from build123d import *

# Parameters (mm, degrees)
F1_DEPTH = 25.4
F2_W     = 19.05
F2_H     = 4.923508
F3_DEPTH = 25.4
F4_R     = 3.175
F5_DEPTH = 12.701
F6_R     = 3.175
F7_DEPTH = 25.4
F8_W     = 19.05
F8_H     = 19.05
F9_DEPTH = 6.35


with BuildPart() as f1:
    # F0 (on Front) → F1 (new body)
    with BuildSketch(Plane.XZ):
        Polygon((-24.8282, 12.7), (-24.8282, 0), (-18.4782, 0), (-18.4782, 6.35), (13.2718, 6.35), (13.2718, 25.4), (-5.7782, 25.4), (-5.7782, 12.7), align=None)
    extrude(amount=F1_DEPTH)

    # F2 (on face) → F3 (cut)
    with BuildSketch(Plane.XY.offset(12.7)):
        with Locations((-15.3032, -22.938246)):
            Rectangle(F2_W, F2_H)
    extrude(amount=-F3_DEPTH, mode=Mode.SUBTRACT)

    # F4 (on face) → F5 (cut, through all)
    with BuildSketch(Plane.XY.offset(12.7)):
        with Locations((-12.1282, -9.525)):
            Circle(F4_R)
    extrude(amount=-F5_DEPTH, mode=Mode.SUBTRACT)

    # F6 (on face) → F7 (cut)
    with BuildSketch(Plane.XY.offset(25.4)):
        with Locations((3.7468, -17.145)):
            Circle(F6_R)
    extrude(amount=-F7_DEPTH, mode=Mode.SUBTRACT)

    # F8 (on face) → F9 (cut)
    with BuildSketch(Plane.XY.offset(25.4)):
        with Locations((3.7468, -15.875)):
            Rectangle(F8_W, F8_H)
    extrude(amount=-F9_DEPTH, mode=Mode.SUBTRACT)


solid = f1.part
Input: part model. Units: mm. Frame: model coordinates. A direction names the side the tool comes from. Give positions to 0.01 mm unless a question says otherwise; leave off trailing zeros. Order: outer loops, then holes, each group sorted by start corner. A loop starts at its lowest first (then second) coordinate and runs counter-clockwise, first axis right, second up. Notation, with made-up numbers: (38.25, 19.5) - (62.25, 19.5) arc R23 ccw to (62.25, 56.5) - close; hole circle Ø3 at (-25.5, 33.25). An arc over 180 degrees is marked (long way). Answer as a JSON object with one key per item and string values. Group by question number.
Q1. Set-up query: faces 5 (the face through (-17, -10, 12.7)), 6 (the face through (4, -3, 25.4)), 7 (the face through (4, -6.35, 22)), 8 (the face through (-18, -20.476, 8)), 9 (the face through (-18.478, -10, 3)). Return all of +Z, -Z, +X, -X, +Y, -Y with unobstructed straight access to the full face (end or side cutting, diameter ignored); none if empty.
Q2. Mould query, pull axis X, two halves, no side actions, for faces 1 (the face through (-15.3, -9.4, 9.6)), 2 (the face through (-22, -10, 0)), 3 (the face through (5.212, -19.962, 12.789)), 4 (the face through (13.272, -13, 14)). Classes: pulls with the +X half, pulls with the -X half, needs draft (parallel to the pull), parting line crosses it, or undercut.
Q3. Line query: probe 1 along Y at (x, z) = (3.5, 9.25); probe 2 along Z at (x, y) = (4, -10.25); probe 3 along X at (y, z) = (-4.75, 16.25). Output: solid intervals per line, ascending.
Q4. Cut plane C-C, the plane x = 7.5. Output: boundary loops of the cut face in (y, z), then the cut area to 3 significant figures.
Q5. Cut plane A-A, the plane x = 2.5. Output: boundary loops of the cut face in (y, z), then the cut area to 3 significant figures.
Q6. First-contact query: pin 1 Ø7 at (x, z) = (7.5, 23) entering from -Y; pin 2 Ø8 at (x, y) = (3, -14.5) entering from -Z; pin 3 Ø8 at (x, y) = (-17.5, -12) entering from +Z. Flat tips, straight axial feed; report the tip coordinate or a pass-through.
Q7. Cut plane B-B, the plane y = -4. Output: boundary loops of the cut face in (x, z), then the cut area to 3 significant figures.
Q8. Cut plane D-D, the plane z = 17. Output: boundary loops of the cut face in (x, y) (3 decimals).
Results:
{
 "1": {"face 5": "+Z, -X, +Y, -Y", "face 6": "+Z, +X, -X, +Y, -Y", "face 7": "+Z, +X, -X, -Y", "face 8": "+Z, -Z, -X, -Y", "face 9": "-Z, +X, +Y, -Y"},
 "2": {"face 1": "undercut", "face 2": "needs draft", "face 3": "undercut", "face 4": "pulls with the +X half"},
 "3": {"probe 1": "-25.4 to -20.31, -13.98 to 0", "probe 2": "6.35 to 19.05", "probe 3": "-5.78 to 13.27"},
 "4": {"outline": "(-25.4, 6.35) - (0, 6.35) - (0, 25.4) - (-6.35, 25.4) - (-6.35, 19.05) - (-25.4, 19.05) - close", "area": "363 mm^2"},
 "5": {"outline": "(-25.4, 6.35) - (-20.06, 6.35) - (-20.06, 19.05) - (-25.4, 19.05) - close; (-14.23, 6.35) - (0, 6.35) - (0, 25.4) - (-6.35, 25.4) - (-6.35, 19.05) - (-14.23, 19.05) - close", "area": "289 mm^2"},
 "6": {"pin 1": "y = -6.35", "pin 2": "z = 6.35", "pin 3": "z = 12.7"},
 "7": {"outline": "(-24.83, 0) - (-18.48, 0) - (-18.48, 6.35) - (13.27, 6.35) - (13.27, 25.4) - (-5.78, 25.4) - (-5.78, 12.7) - (-24.83, 12.7) - close", "area": "524 mm^2"},
 "8": {"outline": "(-5.778, -25.4) - (13.272, -25.4) - (13.272, 0) - (-5.778, 0) - close; hole circle Ø6.35 at (3.747, -17.145)"}
}
